For this review, take the finished solid that the model builds, in its own axes (mm). Face numbers are marked on the shaded views. Round coordinates to 2 decimals unless told otherwise and drop trailing zeros. Write each loop counter-clockwise with the first axis right and the second up, starting at its lowest first coordinate (ties: lowest second). Pieces come first, ordered by that corner, then holes. Notation, with made-up numbers: (-22.5, 47.25) - (-15.5, 47.25) arc R7 ccw to (-15.5, 57.25) - close; hole circle Ø2 at (-23, 26.5). An arc over 180 degrees is marked (long way). Answer in a Markdown table with one row per item. Add a question column.
from build123d import *

# Parameters (mm, degrees)
SKETCH1_W           = 450
SKETCH1_H           = 450
BOSS_EXTRUDE1_DEPTH = 5
BOSS_EXTRUDE2_DEPTH = 7.48
BOSS_EXTRUDE3_DEPTH = 7.48
SKETCH6_W           = 450
SKETCH6_H           = 450
CUT_EXTRUDE1_DEPTH  = 5
SKETCH7_R           = 11
SKETCH7_R_2         = 2.5
CUT_EXTRUDE2_DEPTH  = 10
SKETCH8_R           = 209.3091
SKETCH8_R_2         = 104.5891
CUT_EXTRUDE3_DEPTH  = 10
BOSS_EXTRUDE4_DEPTH = 7.48
SKETCH11_R          = 2.5
CUT_EXTRUDE5_DEPTH  = 10


# Read off the part's stored shape, not the designer's step: Boss-Extrude2
with BuildPart() as part:
    # Sketch1 → Boss-Extrude1 (new body)
    with BuildSketch(Plane(origin=(0, 0, 0), x_dir=(0, 0, -1), z_dir=(1, 0, 0))):
        Rectangle(SKETCH1_W, SKETCH1_H)
    extrude(amount=BOSS_EXTRUDE1_DEPTH)

    # Boss-Extrude2 outline → Boss-Extrude2 (add)
    with BuildSketch(Plane(origin=(5, 0, 0), x_dir=(0, 0, -1), z_dir=(1, 0, 0))):
        with BuildLine():
            Line((-164.971757583, 8.09), (-209.152698388, 8.09))
            ThreePointArc((-209.152698388, 8.09), (-209.3091, 0), (-209.152698388, -8.09))
            Line((-209.152698388, -8.09), (-164.971757583, -8.09))
            ThreePointArc((-164.971757583, -8.09), (-116.792827049, -116.792827049), (-8.09, -164.971757583))
            Line((-8.09, -164.971757583), (-8.09, -209.152698388))
            ThreePointArc((-8.09, -209.152698388), (0, -209.3091), (8.09, -209.152698388))
            Line((8.09, -209.152698388), (8.09, -164.971757583))
            ThreePointArc((8.09, -164.971757583), (116.792827049, -116.792827049), (164.971757583, -8.09))
            Line((164.971757583, -8.09), (209.152698388, -8.09))
            ThreePointArc((209.152698388, -8.09), (209.3091, 0), (209.152698388, 8.09))
            Line((209.152698388, 8.09), (164.971757583, 8.09))
            ThreePointArc((164.971757583, 8.09), (116.792827049, 116.792827049), (8.09, 164.971757583))
            Line((8.09, 164.971757583), (8.09, 209.152698388))
            ThreePointArc((8.09, 209.152698388), (0, 209.3091), (-8.09, 209.152698388))
            Line((-8.09, 209.152698388), (-8.09, 164.971757583))
            ThreePointArc((-8.09, 164.971757583), (-116.792827049, 116.792827049), (-164.971757583, 8.09))
        make_face()
        with BuildLine():
            Line((148.770198629, 8.09), (104.538333308, 8.09))
            ThreePointArc((104.538333308, 8.09), (104.8509, 0), (104.538333308, -8.09))
            Line((104.538333308, -8.09), (148.770198629, -8.09))
            ThreePointArc((148.770198629, -8.09), (105.351839329, -105.351839329), (8.09, -148.770198629))
            Line((8.09, -148.770198629), (8.09, -104.538333308))
            ThreePointArc((8.09, -104.538333308), (0, -104.8509), (-8.09, -104.538333308))
            Line((-8.09, -104.538333308), (-8.09, -148.770198629))
            ThreePointArc((-8.09, -148.770198629), (-105.351839329, -105.351839329), (-148.770198629, -8.09))
            Line((-148.770198629, -8.09), (-104.538333308, -8.09))
            ThreePointArc((-104.538333308, -8.09), (-104.8509, 0), (-104.538333308, 8.09))
            Line((-104.538333308, 8.09), (-148.770198629, 8.09))
            ThreePointArc((-148.770198629, 8.09), (-105.351839329, 105.351839329), (-8.09, 148.770198629))
            Line((-8.09, 148.770198629), (-8.09, 104.538333308))
            ThreePointArc((-8.09, 104.538333308), (0, 104.8509), (8.09, 104.538333308))
            Line((8.09, 104.538333308), (8.09, 148.770198629))
            ThreePointArc((8.09, 148.770198629), (105.351839329, 105.351839329), (148.770198629, 8.09))
        make_face(mode=Mode.SUBTRACT)
    extrude(amount=BOSS_EXTRUDE2_DEPTH)

    # Sketch5 → Boss-Extrude3 (add)
    with BuildSketch(Plane(origin=(5, 0, 0), x_dir=(0, 0, -1), z_dir=(1, 0, 0))):
        with BuildLine():
            Line((-19.319547743, 8.09), (-104.275748565, 8.09))
            ThreePointArc((-104.275748565, 8.09), (-104.5891, 0), (-104.275748565, -8.09))
            Line((-104.275748565, -8.09), (-19.319547743, -8.09))
            ThreePointArc((-19.319547743, -8.09), (0, -20.945), (19.319547743, -8.09))
            Line((19.319547743, -8.09), (104.275748565, -8.09))
            ThreePointArc((104.275748565, -8.09), (104.5891, 0), (104.275748565, 8.09))
            Line((104.275748565, 8.09), (19.319547743, 8.09))
            ThreePointArc((19.319547743, 8.09), (0, 20.945), (-19.319547743, 8.09))
        make_face()
    extrude(amount=BOSS_EXTRUDE3_DEPTH)

    # Sketch6 → Cut-Extrude1 (cut)
    with BuildSketch(Plane.ZY):
        Rectangle(SKETCH6_W, SKETCH6_H)
    extrude(amount=-CUT_EXTRUDE1_DEPTH, mode=Mode.SUBTRACT)


with BuildPart() as cut_extrude1_piece_1:
    # of the separate pieces the step leaves, piece 1, a body of its own (cut_extrude1_pieces)
    add(part.part.solids().sort_by_distance((5, 209.152698388, 8.09))[0])


with BuildPart() as cut_extrude1_piece_2:
    # of the separate pieces the step leaves, piece 2, a body of its own (cut_extrude1_pieces)
    add(part.part.solids().sort_by_distance((5, 8.09, -104.275748565))[0])


with BuildPart() as cut_extrude2_tool:
    # Sketch7 → Cut-Extrude2 (new body)
    with BuildSketch(Plane(origin=(12.48, 0, 0), x_dir=(0, 0, -1), z_dir=(1, 0, 0))):
        Circle(SKETCH7_R)
        with Locations((-183.1891, 0)):
            Circle(SKETCH7_R_2)
        with Locations((-130.9659, 0)):
            Circle(SKETCH7_R_2)
        with Locations((0, -183.1891)):
            Circle(SKETCH7_R_2)
        with Locations((0, -130.9659)):
            Circle(SKETCH7_R_2)
        with Locations((183.1891, 0)):
            Circle(SKETCH7_R_2)
        with Locations((52.3, 0)):
            Circle(SKETCH7_R_2)
        with Locations((-52.295, 0)):
            Circle(SKETCH7_R_2)
        with Locations((0, 183.1891)):
            Circle(SKETCH7_R_2)
        with Locations((0, 130.9659)):
            Circle(SKETCH7_R_2)
        with BuildLine():
            Line((-3, 13.8), (-3, 10.583005244))
            ThreePointArc((-3, 10.583005244), (0, 11), (3, 10.583005244))
            Line((3, 10.583005244), (3, 13.8))
            Line((3, 13.8), (-3, 13.8))
        make_face()
        with BuildLine():
            ThreePointArc((3, -10.583005244), (0, -11), (-3, -10.583005244))
            Line((-3, -10.583005244), (-3, -13.8))
            Line((-3, -13.8), (3, -13.8))
            Line((3, -13.8), (3, -10.583005244))
        make_face()
        with Locations((130.9659, 0)):
            Circle(SKETCH7_R_2)
    extrude(amount=-CUT_EXTRUDE2_DEPTH)


with BuildPart() as cut_extrude1_piece_1_1:
    add(cut_extrude1_piece_1.part)

    # Cut-Extrude2: cut by cut_extrude2_tool
    add(cut_extrude2_tool.part, mode=Mode.SUBTRACT)

    # Sketch8 → Cut-Extrude3 (cut)
    with BuildSketch(Plane(origin=(12.48, 0, 0), x_dir=(0, 0, -1), z_dir=(1, 0, 0))):
        Circle(SKETCH8_R)
        Circle(SKETCH8_R_2, mode=Mode.SUBTRACT)
    extrude(amount=-CUT_EXTRUDE3_DEPTH, mode=Mode.SUBTRACT)


with BuildPart() as cut_extrude1_piece_2_1:
    add(cut_extrude1_piece_2.part)

    # Cut-Extrude2: cut by cut_extrude2_tool
    add(cut_extrude2_tool.part, mode=Mode.SUBTRACT)

    # Sketch9 → Boss-Extrude4 (add)
    with BuildSketch(Plane(origin=(12.48, 0, 0), x_dir=(0, 0, -1), z_dir=(1, 0, 0))):
        with BuildLine():
            Line((-94.350447256, 45.131728766), (-30.192291033, 8.09))
            Line((-30.192291033, 8.09), (-19.319547743, 8.09))
            ThreePointArc((-19.319547743, 8.09), (0, 20.945), (19.319547743, 8.09))
            Line((19.319547743, 8.09), (30.192291033, 8.09))
            Line((30.192291033, 8.09), (94.350447256, 45.131728766))
            ThreePointArc((94.350447256, 45.131728766), (90.576817559, 52.29455), (86.260447256, 59.144019799))
            Line((86.260447256, 59.144019799), (22.102291033, 22.102291033))
            Line((22.102291033, 22.102291033), (59.144019799, 86.260447256))
            ThreePointArc((59.144019799, 86.260447256), (52.29455, 90.576817559), (45.131728766, 94.350447256))
            Line((45.131728766, 94.350447256), (8.09, 30.192291033))
            Line((8.09, 30.192291033), (8.09, 104.275748565))
            ThreePointArc((8.09, 104.275748565), (0, 104.5891), (-8.09, 104.275748565))
            Line((-8.09, 104.275748565), (-8.09, 30.192291033))
            Line((-8.09, 30.192291033), (-45.131728766, 94.350447256))
            ThreePointArc((-45.131728766, 94.350447256), (-52.29455, 90.576817559), (-59.144019799, 86.260447256))
            Line((-59.144019799, 86.260447256), (-22.102291033, 22.102291033))
            Line((-22.102291033, 22.102291033), (-86.260447256, 59.144019799))
            ThreePointArc((-86.260447256, 59.144019799), (-90.576817559, 52.29455), (-94.350447256, 45.131728766))
        make_face()
        with BuildLine():
            ThreePointArc((19.319547743, -8.09), (0, -20.945), (-19.319547743, -8.09))
            Line((-19.319547743, -8.09), (-30.192291033, -8.09))
            Line((-30.192291033, -8.09), (-94.350447256, -45.131728766))
            ThreePointArc((-94.350447256, -45.131728766), (-90.576817559, -52.29455), (-86.260447256, -59.144019799))
            Line((-86.260447256, -59.144019799), (-22.102291033, -22.102291033))
            Line((-22.102291033, -22.102291033), (-59.144019799, -86.260447256))
            ThreePointArc((-59.144019799, -86.260447256), (-52.29455, -90.576817559), (-45.131728766, -94.350447256))
            Line((-45.131728766, -94.350447256), (-8.09, -30.192291033))
            Line((-8.09, -30.192291033), (-8.09, -104.275748565))
            ThreePointArc((-8.09, -104.275748565), (0, -104.5891), (8.09, -104.275748565))
            Line((8.09, -104.275748565), (8.09, -30.192291033))
            Line((8.09, -30.192291033), (45.131728766, -94.350447256))
            ThreePointArc((45.131728766, -94.350447256), (52.29455, -90.576817559), (59.144019799, -86.260447256))
            Line((59.144019799, -86.260447256), (22.102291033, -22.102291033))
            Line((22.102291033, -22.102291033), (86.260447256, -59.144019799))
            ThreePointArc((86.260447256, -59.144019799), (90.576817559, -52.29455), (94.350447256, -45.131728766))
            Line((94.350447256, -45.131728766), (30.192291033, -8.09))
            Line((30.192291033, -8.09), (19.319547743, -8.09))
        make_face()
    extrude(amount=-BOSS_EXTRUDE4_DEPTH)

    # Sketch11 → Cut-Extrude5 (cut)
    with BuildSketch(Plane(origin=(12.48, 0, 0), x_dir=(0, 0, -1), z_dir=(1, 0, 0))):
        with Locations((-52.295, 0)):
            Circle(SKETCH11_R)
        with Locations((-45.288798491, 26.1475)):
            Circle(SKETCH11_R)
        with Locations((-26.1475, 45.288798491)):
            Circle(SKETCH11_R)
        with Locations((0, 52.295)):
            Circle(SKETCH11_R)
        with Locations((26.1475, 45.288798491)):
            Circle(SKETCH11_R)
        with Locations((45.288798491, 26.1475)):
            Circle(SKETCH11_R)
        with Locations((52.295, 0)):
            Circle(SKETCH11_R)
        with Locations((45.288798491, -26.1475)):
            Circle(SKETCH11_R)
        with Locations((26.1475, -45.288798491)):
            Circle(SKETCH11_R)
        with Locations((0, -52.295)):
            Circle(SKETCH11_R)
        with Locations((-26.1475, -45.288798491)):
            Circle(SKETCH11_R)
        with Locations((-45.288798491, -26.1475)):
            Circle(SKETCH11_R)
    extrude(amount=-CUT_EXTRUDE5_DEPTH, mode=Mode.SUBTRACT)


solid = cut_extrude1_piece_2_1.part
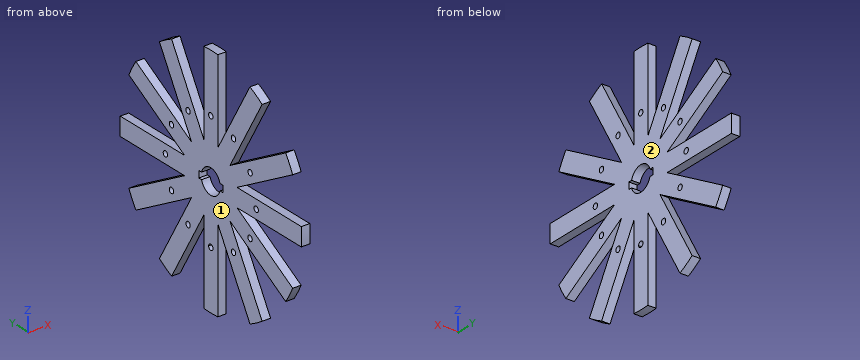
Q1. Add section D-D on z = -34.5. State the section outline as (x, y) points.
Q2. Draft analysis for pull direction X (two halves, no side actions). For the marked faces 1 and 2, state which applies: released by +X, released by -X, zero draft, split by the parting line, or undercut.
Q3. To check wall thickness, follow probe 1 along Y at (x, z) = (10.25, -41); probe 2 along Z at (x, y) = (7, 36); probe 3 along Y at (x, z) = (7.75, 54.5). State the ranges of each line that lie inside material, in increasing order.
Q4. Insertion check: pin 1 Ø2 at (x, y) = (9, -60) entering from +Z; pin 2 Ø2.5 at (x, y) = (9, 11.5) entering from -Z; pin 3 Ø2 at (x, y) = (7.5, 16) entering from -Z. Each pin has a flat end and moves straight along its axis. Give the tip position at first contact, or say it passes through.
Q5. Add section C-C on y = -83. State the section outline as (x, z) points, then the cut area to 3 significant figures.
Q6. Add section B-B on z = 0. State the section outline as (x, y) points (3 decimals).
Q7. Add section A-A on y = 0. State the section outline as (x, z) points (3 decimals), then the cut area to 3 significant figures.
Answer sheet:
| question | item | result |
|---|---|---|
| 1 | outline | (5, -75.94) - (12.48, -75.94) - (12.48, -43.58) - (5, -43.58) - close; (5, -29.26) - (12.48, -29.26) - (12.48, -10.58) - (5, -10.58) - close; (5, -8.09) - (12.48, -8.09) - (12.48, 8.09) - (5, 8.09) - close; (5, 10.58) - (12.48, 10.58) - (12.48, 29.26) - (5, 29.26) - close; (5, 43.58) - (12.48, 43.58) - (12.48, 75.94) - (5, 75.94) - close |
| 2 | face 1 | released by -X |
| 2 | face 2 | released by +X |
| 3 | probe 1 | y = -87.19 to -54.83, -33.01 to -14.33, -8.09 to 8.09, 14.33 to 33.01, 54.83 to 87.19 |
| 3 | probe 2 | z = -78.53 to -46.17, -30.13 to -11.44, -8.09 to 8.09, 11.44 to 30.13, 46.17 to 78.53 |
| 3 | probe 3 | y = -89.27 to -78.22, -40.81 to -22.12, -8.09 to -1.18, 1.18 to 8.09, 22.12 to 40.81, 78.22 to 89.27 |
| 4 | pin 1 | stops at z = 86.36 |
| 4 | pin 2 | stops at z = -38.26 |
| 4 | pin 3 | stops at z = -45.62 |
| 5 | outline | (5, -57.26) - (12.48, -57.26) - (12.48, -38.58) - (5, -38.58) - close; (5, -8.09) - (12.48, -8.09) - (12.48, 8.09) - (5, 8.09) - close; (5, 38.58) - (12.48, 38.58) - (12.48, 57.26) - (5, 57.26) - close |
| 5 | area | 401 mm² |
| 6 | outline | (5, -104.589) - (12.48, -104.589) - (12.48, -54.795) - (5, -54.795) - close; (5, -49.795) - (12.48, -49.795) - (12.48, -13.8) - (5, -13.8) - close; (5, 13.8) - (12.48, 13.8) - (12.48, 49.795) - (5, 49.795) - close; (5, 54.795) - (12.48, 54.795) - (12.48, 104.589) - (5, 104.589) - close |
| 7 | outline | (5, -104.589) - (12.48, -104.589) - (12.48, -54.8) - (5, -54.8) - close; (5, -49.795) - (12.48, -49.795) - (12.48, -11) - (5, -11) - close; (5, 11) - (12.48, 11) - (12.48, 49.795) - (5, 49.795) - close; (5, 54.795) - (12.48, 54.795) - (12.48, 104.589) - (5, 104.589) - close |
| 7 | area | 1,330 mm² |
